Build history of the part. All positions in model axes, mm. Give positions to 0.01 mm unless a question says otherwise; leave off trailing zeros. Order: outer loops, then holes, each group sorted by start corner. A loop starts at its lowest first (then second) coordinate and runs counter-clockwise, first axis right, second up. Notation, with made-up numbers: M 43.25,44.5 L 59.25,44.5 A26 ccw 59.25,59.5 Z; hole C 23.5,87.5 d11. An arc over 180 degrees is marked long. One line per item, written item: value.
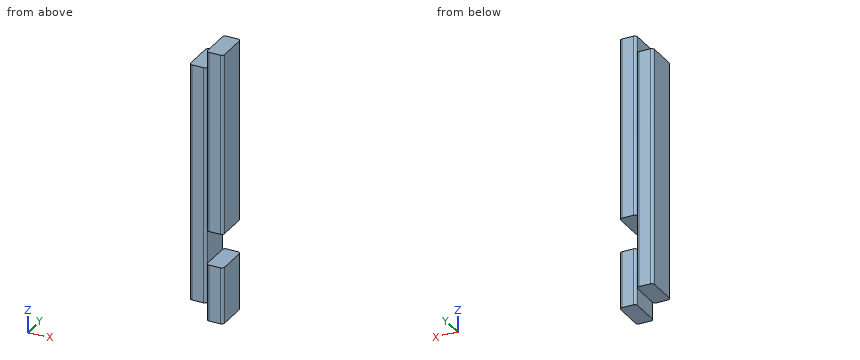
from build123d import *

# Parameters (mm, degrees)
F1_DEPTH = 304.8
F2_DEPTH = 285.75
F3_DEPTH = 19.05
F4_W     = 19.05
F4_H     = 38.1
F5_DEPTH = 38.101


# Not quite as in the source:
# - a feature names something its author has since deleted; it is built from what else it names


with BuildPart() as f1:
    # F0 (on Top) → F1 (new body)
    with BuildSketch(Plane.XY):
        with BuildLine():
            Line((19.05, 34.9504), (19.05, 3.1496))
            ThreePointArc((19.05, 3.1496), (19.972496482, 0.922496482), (22.1996, 0))
            Line((22.1996, 0), (34.9504, 0))
            ThreePointArc((34.9504, 0), (37.177503518, 0.922496482), (38.1, 3.1496))
            Line((38.1, 3.1496), (38.1, 34.9504))
            ThreePointArc((38.1, 34.9504), (37.177503518, 37.177503518), (34.9504, 38.1))
            Line((34.9504, 38.1), (22.1996, 38.1))
            ThreePointArc((22.1996, 38.1), (19.972496482, 37.177503518), (19.05, 34.9504))
        make_face()
    extrude(amount=F1_DEPTH)

    # F0 (on Top) → F2 (join)
    with BuildSketch(Plane.XY):
        with BuildLine():
            ThreePointArc((0, 3.1496), (0.922496482, 0.922496482), (3.1496, 0))
            Line((3.1496, 0), (15.9004, 0))
            ThreePointArc((15.9004, 0), (18.127503518, 0.922496482), (19.05, 3.1496))
            Line((19.05, 3.1496), (19.05, 34.9504))
            ThreePointArc((19.05, 34.9504), (18.127503518, 37.177503518), (15.9004, 38.1))
            Line((15.9004, 38.1), (3.1496, 38.1))
            ThreePointArc((3.1496, 38.1), (0.922496482, 37.177503518), (0, 34.9504))
            Line((0, 34.9504), (0, 3.1496))
        make_face()
        with BuildLine():
            Line((19.05, 34.9504), (19.05, 3.1496))
            ThreePointArc((19.05, 3.1496), (19.972496482, 0.922496482), (22.1996, 0))
            Line((22.1996, 0), (34.9504, 0))
            ThreePointArc((34.9504, 0), (37.177503518, 0.922496482), (38.1, 3.1496))
            Line((38.1, 3.1496), (38.1, 34.9504))
            ThreePointArc((38.1, 34.9504), (37.177503518, 37.177503518), (34.9504, 38.1))
            Line((34.9504, 38.1), (22.1996, 38.1))
            ThreePointArc((22.1996, 38.1), (19.972496482, 37.177503518), (19.05, 34.9504))
        make_face()
    extrude(amount=F2_DEPTH)

    # F0 (on Top) → F3 (cut)
    with BuildSketch(Plane.XY):
        with BuildLine():
            ThreePointArc((0, 3.1496), (0.922496482, 0.922496482), (3.1496, 0))
            Line((3.1496, 0), (15.9004, 0))
            ThreePointArc((15.9004, 0), (18.127503518, 0.922496482), (19.05, 3.1496))
            Line((19.05, 3.1496), (19.05, 34.9504))
            ThreePointArc((19.05, 34.9504), (18.127503518, 37.177503518), (15.9004, 38.1))
            Line((15.9004, 38.1), (3.1496, 38.1))
            ThreePointArc((3.1496, 38.1), (0.922496482, 37.177503518), (0, 34.9504))
            Line((0, 34.9504), (0, 3.1496))
        make_face()
    extrude(amount=F3_DEPTH, mode=Mode.SUBTRACT)

    # F4 (on face) → F5 (cut, through all)
    with BuildSketch(Plane.XZ):
        with Locations((28.575, 82.55)):
            Rectangle(F4_W, F4_H)
    extrude(amount=-F5_DEPTH, mode=Mode.SUBTRACT)


solid = f1.part
1) Saw through at A-A, the plane x = 27.5. Write the cut outline in (y, z).
Check values:
outline: M 0,0 L 38.1,0 L 38.1,63.5 L 0,63.5 Z; M 0,101.6 L 38.1,101.6 L 38.1,304.8 L 0,304.8 Z
2) Pin check, flat tips, straight feed: pin 1 (9.5 mm diameter, centred on y = 12, z = 294.5, fed in from -X); pin 2 (9.5 mm diameter, centred on x = 9.5, y = 12, fed in from +Z); pin 3 (5.5 mm diameter, centred on x = 11, y = 10.5, fed in from -Z). Stop position of each tip, or through.
Check values:
pin 1: x = 19.05
pin 2: z = 285.75
pin 3: z = 19.05
3) Saw through at D-D, the plane x = 12.5. Write the cut outline in (y, z), then the cut area to 3 significant figures.
Check values:
outline: M 0,19.05 L 38.1,19.05 L 38.1,285.75 L 0,285.75 Z
area: 10,200 mm^2
4) Drill centre lines: probe 1 along Z at (x, y) = (34.5, 4); probe 2 along Z at (x, y) = (7.5, 16.5); probe 3 along Y at (x, z) = (16, 189). Where is each one in solid material? Low to high. Write a range as from..to.
Check values:
probe 1: 0..63.5, 101.6..304.8
probe 2: 19.05..285.75
probe 3: 0..38.1
5) Saw through at C-C, the plane z = 97.5. Write the cut outline in (x, y).
Check values:
outline: M 0,3.15 A3.15 ccw 3.15,0 L 15.9,0 A3.15 ccw 19.05,3.15 L 19.05,34.95 A3.15 ccw 15.9,38.1 L 3.15,38.1 A3.15 ccw 0,34.95 Z
6) Saw through at B-B, the plane y = 12. Write the cut outline in (x, z).
Check values:
outline: M 0,19.05 L 19.05,19.05 L 19.05,0 L 38.1,0 L 38.1,63.5 L 19.05,63.5 L 19.05,101.6 L 38.1,101.6 L 38.1,304.8 L 19.05,304.8 L 19.05,285.75 L 0,285.75 Z
